```python
from build123d import *

# Parameters (mm, degrees)
SKETCH1_R           = 12.7
BOSS_EXTRUDE1_DEPTH = 12.7


with BuildPart() as part:
    # Sketch1 → Boss-Extrude1 (new body)
    with BuildSketch(Plane(origin=(0, 0, 0), x_dir=(1, 0, 0), z_dir=(0, 1, 0))):
        with BuildLine():
            ThreePointArc((-177.79300078, -55.798766176), (-170.27365382, -37.758748247), (-152.16762701, -30.399766064))
            Line((-152.16762701, -30.399766064), (152.618374551, -33.104233568))
            ThreePointArc((152.618374551, -33.104233568), (170.43301871, -40.622580641), (177.79300078, -58.50323368))
            Line((177.79300078, -58.50323368), (177.79300078, -500))
            Line((177.79300078, -500), (500, -177.79300078))
            Line((500, -177.79300078), (500, 500))
            Line((500, 500), (177.79300078, 177.79300078))
            Line((177.79300078, 177.79300078), (177.79300078, 55.798766176))
            ThreePointArc((177.79300078, 55.798766176), (170.27365382, 37.758748247), (152.16762701, 30.399766064))
            Line((152.16762701, 30.399766064), (12.711649925, 31.637205305))
            Line((12.711649925, 31.637205305), (12.711649925, 326.507694892))
            ThreePointArc((12.711649925, 326.507694892), (0, 380.747448982), (-12.711649925, 326.507694892))
            Line((-12.711649925, 326.507694892), (-12.711649925, 31.862794695))
            Line((-12.711649925, 31.862794695), (-152.618374551, 33.104233568))
            ThreePointArc((-152.618374551, 33.104233568), (-170.43301871, 40.62258064), (-177.79300078, 58.50323368))
            Line((-177.79300078, 58.50323368), (-177.79300078, 500))
            Line((-177.79300078, 500), (-500, 177.79300078))
            Line((-500, 177.79300078), (-500, -500))
            Line((-500, -500), (-177.79300078, -177.79300078))
            Line((-177.79300078, -177.79300078), (-177.79300078, -55.798766176))
        make_face()
        Circle(SKETCH1_R, mode=Mode.SUBTRACT)
    extrude(amount=BOSS_EXTRUDE1_DEPTH)


solid = part.part
```
Check sheet for the modelled part. Datum: model origin and axes. Units: mm. A direction names the side the tool comes from. Round coordinates to 2 decimals unless told otherwise and drop trailing zeros. Write each loop counter-clockwise with the first axis right and the second up, starting at its lowest first coordinate (ties: lowest second). Pieces come first, ordered by that corner, then holes. Notation, with made-up numbers: (46, 86.5) -> (93, 86.5) arc R27 ccw to (93, 115.5) -> close; hole circle Ø10 at (31, 84.25). An arc over 180 degrees is marked (long way). Put each result on its own line as item: value.
(1) Sectioned sample at D-D (x = -214). Enter the section's corners in (y, z).
Values found:
outline: (0, -463.79) -> (12.7, -463.79) -> (12.7, 214) -> (0, 214) -> close
(2) Tool access check on faces 1 (the face through (170.472, 6.261, -37.958)), 2 (the face through (-118, 12.7, -7)), 3 (the face through (-170.472, 6.261, 37.958)). Record the directions out of +Z, -Z, +X, -X, +Y, -Y that give a thin tool (end or side, any length) a straight path to the whole face; none if there is none.
Values found:
face 1: -Z, +Y, -Y
face 2: +Z, -Z, +X, -X, +Y
face 3: +Z, +Y, -Y
(3) Sectioned sample at B-B (z = 0). Enter the section's corners in (x, y).
Values found:
outline: (-500, 0) -> (-12.7, 0) -> (-12.7, 12.7) -> (-500, 12.7) -> close; (12.7, 0) -> (500, 0) -> (500, 12.7) -> (12.7, 12.7) -> close
(4) Go/stop test with flat-tipped pins: pin 1 Ø4 at (y, z) = (4, 248.5) entering from +X; pin 2 Ø3 at (x, y) = (-40.5, 9) entering from +Z; pin 3 Ø6 at (x, y) = (235.5, 4.5) entering from -Z. Record where each tip stops, or that it passes through.
Values found:
pin 1: stops at x = 431.29
pin 2: stops at z = 31.4
pin 3: stops at z = -238.5
(5) Material ranges on line 1 (X direction, y = 5.25, z = 0); line 2 (Z direction, x = 149.5, y = 7.75); line 3 (Z direction, x = -22, y = 9.25), recorded low to high.
Values found:
line 1: x = -500 to -12.7, 12.7 to 500
line 2: z = -30.42 to 33.08
line 3: z = -370.43 to -333.85, -31.95 to 31.55
(6) Mould release check, pull along X, two halves, no side actions. Record for faces 4 (the face through (170.24, 6.26, 40.43)), 5 (the face through (-118, 0, -7)), 6 (the face through (-336.641, 6.261, -341.152)): released by +X, released by -X, zero draft, split by the parting line, or undercut.
Values found:
face 4: undercut
face 5: zero draft
face 6: released by -X
(7) Sectioned sample at C-C (y = 5.75). Enter the section's corners in (x, z), plus the area to 3 significant figures.
Values found:
outline: (-500, -177.79) -> (-177.79, -500) -> (-177.79, -58.5) arc R25.4 cw to (-152.62, -33.1) -> (-12.71, -31.86) -> (-12.71, -326.51) arc R28.61 ccw (long way) to (12.71, -326.51) -> (12.71, -31.64) -> (152.17, -30.4) arc R25.4 cw to (177.79, -55.8) -> (177.79, -177.79) -> (500, -500) -> (500, 177.79) -> (177.79, 500) -> (177.79, 58.5) arc R25.4 cw to (152.62, 33.1) -> (-152.17, 30.4) arc R25.4 cw to (-177.79, 55.8) -> (-177.79, 177.79) -> (-500, 500) -> close; hole circle Ø25.4 at (0, 0)
area: 469,000 mm^2
(8) Sectioned sample at A-A (x = 0). Enter the section's corners in (y, z).
Values found:
outline: (0, -380.75) -> (12.7, -380.75) -> (12.7, -12.7) -> (0, -12.7) -> close; (0, 12.7) -> (12.7, 12.7) -> (12.7, 31.75) -> (0, 31.75) -> close
